CAD build for the part. Positions are in the model's coordinates, mm. Face numbers are marked on the shaded views. A direction names the side the tool comes from. Coordinates: 2 decimals unless noted, no trailing zeros. Loops run counter-clockwise (first coordinate to the right, second up) from the corner with the lowest first, then second, coordinate; pieces in that order, holes last.
1) Which spindle directions (+Z, -Z, +X, -X, +Y, -Y) get a long thin tool onto all of the face, cutting with end or side? Do the marked faces 1, 2 and 3. Say none if no direction does.
2) Wall check: line 1 along X through (y, z) = (-12, 0); line 2 along Z through (x, y) = (5.5, 8.5); line 3 along Y through (x, z) = (21.5, -6). Give the ranges that are in metal, low to high.
3) Saw through at D-D, the plane y = -12.5. Write the cut outline in (x, z), and give its area (3 significant figures).
4) Saw through at B-B, the plane z = -15.5. Write the cut outline in (x, y).
5) Two-plate mould, pull along X, no slides. Class the marked faces 4, 5 and 6: +X half, -X half, draft (parallel to the pull), parting line (faces both ways), or undercut.
6) Pin check, flat tips, straight feed: pin 1 Ø8 at (x, y) = (-32, 7.5) entering from -Z; pin 2 Ø5 at (x, y) = (12.5, 12) entering from -Z; pin 3 Ø1 at (x, z) = (8, -12.5) entering from -Y. Stop position of each tip, or through.
7) Saw through at A-A, the plane x = 0. Write the cut outline in (y, z), and give its area (4 significant figures).
8) Saw through at C-C, the plane y = 9. Write the cut outline in (x, z), and give its area (3 significant figures).
```python
from build123d import *

# Parameters (mm, degrees)
SKIZZE1_R                          = 50
AUFSATZ_LINEAR_AUSTRAGEN1_DEPTH    = 20
SKIZZE2_R                          = 40
SCHNITT_LINEAR_AUSTRAGEN1_DEPTH    = 5
SKIZZE3_R                          = 7.5
AUFSATZ_LINEAR_AUSTRAGEN2_DEPTH    = 59.5
SKALIEREN1_SCALE                   = 0.75
K_RPER_VERSCHIEBEN_KOPIEREN1_ANGLE = 120


with BuildPart() as part:
    # Skizze1 → Aufsatz-Linear austragen1 (new, symmetric)
    with BuildSketch(Plane(origin=(0, 0, 0), x_dir=(0, 1, 0), z_dir=(0, 0, 1))):
        with Locations(Location((0, 0, 0), (0, 0, 270))):
            Circle(SKIZZE1_R)
    extrude(amount=AUFSATZ_LINEAR_AUSTRAGEN1_DEPTH, both=True)

    # Skizze2 → Schnitt-Linear austragen1 (cut)
    with BuildSketch(Plane.XY.offset(20)):
        Circle(SKIZZE2_R)
    extrude(amount=-SCHNITT_LINEAR_AUSTRAGEN1_DEPTH, mode=Mode.SUBTRACT)

    # Skizze3 → Aufsatz-Linear austragen2 (add, symmetric)
    with BuildSketch(Plane(origin=(0, 0, 0), x_dir=(-1, 0, 0), z_dir=(0, 1, 0))):
        with Locations(Location((0, 0, 0), (0, 0, 270))):
            Circle(SKIZZE3_R)
    extrude(amount=AUFSATZ_LINEAR_AUSTRAGEN2_DEPTH, both=True)


with BuildPart() as part_1:
    # Skalieren1: scaled about (4.8248e-05, 1e-09, -1.504015825)
    add(part.part.scale(SKALIEREN1_SCALE).moved(Location((1.2062e-05, 0, -0.376003956))))


with BuildPart() as part_2:
    # Körper-Verschieben/Kopieren1: moved
    add(part_1.part.rotate(Axis((0, 0, 0), (0.5773502691896928, 0.5773502691894897, -0.5773502691896948)), K_RPER_VERSCHIEBEN_KOPIEREN1_ANGLE))


solid = part_2.part
```
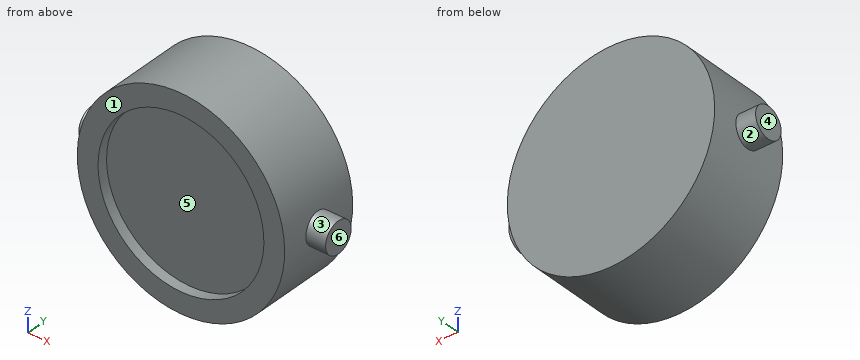
Data:
1. face 1: +Z, -Z, +X, -X, -Y
1. face 2: -X
1. face 3: +X
2. line 1: x = -37.5 to -30, 30 to 37.5
2. line 2: z = -37.09 to 37.09
2. line 3: y = -10.87 to 15.38
3. outline: circle Ø75 at (0, 0); hole circle Ø60 at (0, 0)
3. area: 1,590 mm2
4. outline: (-34.15, -14.62) - (-25.69, -14.62) - (-25.69, -10.87) - (25.69, -10.87) - (25.69, -14.62) - (34.15, -14.62) - (34.15, 15.38) - (-34.15, 15.38) - close
5. face 4: -X half
5. face 5: undercut
5. face 6: +X half
6. pin 1: stops at z = -24.94
6. pin 2: stops at z = -36.14
6. pin 3: stops at y = -10.87
7. outline: (-14.62, -37.5) - (15.38, -37.5) - (15.38, 37.5) - (-14.62, 37.5) - (-14.62, 30) - (-10.87, 30) - (-10.87, -30) - (-14.62, -30) - close
7. area: 2,025 mm2
8. outline: circle Ø75 at (0, 0)
8. area: 4,420 mm2
